Design review of the part built by this model. Coordinates are the model's own, in mm. Face numbers are marked on the shaded views. A direction names the side the tool comes from. Round coordinates to 2 decimals unless told otherwise and drop trailing zeros. Order: outer loops, then holes, each group sorted by start corner. A loop starts at its lowest first (then second) coordinate and runs counter-clockwise, first axis right, second up.
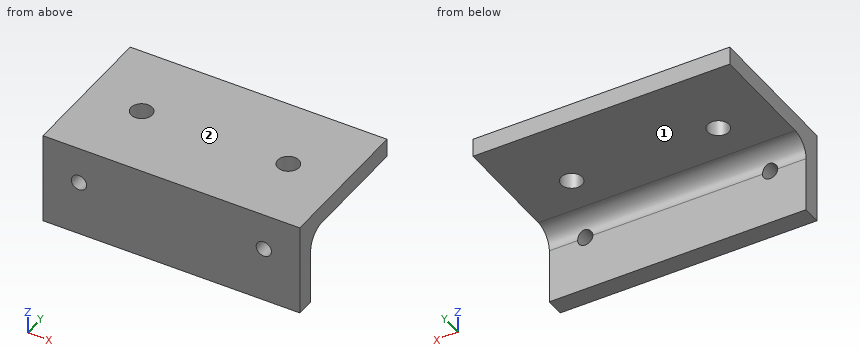
Autodesk Inventor part; units mm, degrees
ref_plane "YZ Plane" through (0, 0, 0) normal (1, 0, 0) x (0, 1, 0)
ref_plane "XZ Plane" through (0, 0, 0) normal (0, 1, 0) x (-1, 0, 0)
ref_plane "XY Plane" through (0, 0, 0) normal (0, 0, 1) x (1, 0, 0)
sketch "Sketch1" plane through (0, 0, 0) normal (1, 0, 0) x (0, 1, 0)
  line L0 (0, 0) -> (25.4, 0)
  line L1 (25.4, 0) -> (25.4, -3.175)
  line L2 (25.4, -3.175) -> (3.175, -3.175)
  line L3 (3.175, -3.175) -> (3.175, -15.875)
  line L4 (3.175, -15.875) -> (0, -15.875)
  line L5 (0, -15.875) -> (0, 0)
  dimension "d0" = 25.4
  dimension "d2" = 3.175
  dimension "d21" = 15.875
extrude "Extrusion1" add sketch "Sketch1" along normal mid plane 44.45
fillet "Fillet1" radius 3.175 1 edges at (0, 3.175, -3.175)
sketch "Sketch2" plane through (-22.225, 0, -15.875) normal (0, -1, 0) x (1, 0, 0)
  line L0 (38.225, 9.525) -> (6.225, 9.525) construction
  line L1 (0, 15.875) -> (44.45, 15.875) construction
  point P0 (22.225, 15.875)
  point P1 (22.225, 9.525)
  point P2 (22.225, 15.875)
  dimension "d6" = 6.35
  dimension "d7" = 32
hole "Hole1" at (16, 0, -6.35) at (-16, 0, -6.35) direction (0, 1, 0) diameter 2.6416 end through all
sketch "Sketch3" plane through (-22.225, 0, 0) normal (0, 0, 1) x (1, 0, 0)
  line L0 (0, 0) -> (44.45, 0) construction
  line L1 (0, 25.4) -> (44.45, 25.4) construction
  line L2 (34.925, 12.7) -> (9.525, 12.7) construction
  point P0 (22.225, 0)
  point P1 (22.225, 0)
  point P2 (22.225, 12.7)
  point P3 (22.225, 0)
  dimension "d15" = 25.4
  dimension "d22" = 12.7
hole "Hole2" at (12.7, 12.7, 0) at (-12.7, 12.7, 0) direction (0, 0, -1) diameter 3.683 end through all
properties part number "GP7-005" material "Aluminum 6061"
1) To check wall thickness, follow line 1 along X through (y, z) = (1.2, -6.35) (3 decimals); line 2 along X through (y, z) = (12.7, -0.95) (1 decimal); line 3 along Y through (x, z) = (12.7, -1.55). State the ranges of each line that lie inside material, in increasing order.
Results:
line 1: x = -22.225 to -17.321, -14.679 to 14.679, 17.321 to 22.225
line 2: x = -22.2 to -14.5, -10.9 to 10.9, 14.5 to 22.2
line 3: y = 0 to 10.86, 14.54 to 25.4
2) Clearance check with flat-ended pins moving along their axes: P1, Ø8, axis at y = 22, z = -11, coming from the +X side; P2, Ø3, axis at x = 16, z = -6.35, coming from the +Y side; P3, Ø1.5, axis at x = 14, y = 10, coming from the -Z side (3 decimals). State where each tip first meets the part, or that it passes through.
Results:
P1: passes through
P2: stops at y = 3.55
P3: stops at z = -3.175
3) Take a section at A-A on y = 12.7. Give the boundary of the cut face in (x, z) (1 decimal).
Results:
outline: (-22.2, -3.2) - (-14.5, -3.2) - (-14.5, 0) - (-22.2, 0) - close; (-10.9, -3.2) - (10.9, -3.2) - (10.9, 0) - (-10.9, 0) - close; (14.5, -3.2) - (22.2, -3.2) - (22.2, 0) - (14.5, 0) - close
4) Take a section at D-D on y = 2. Give the boundary of the cut face in (x, z) (3 decimals).
Results:
outline: (-22.225, -15.875) - (22.225, -15.875) - (22.225, 0) - (-22.225, 0) - close; hole circle Ø2.642 at (-16, -6.35); hole circle Ø2.642 at (16, -6.35)
5) Take a section at C-C on x = 5. Give the boundary of the cut face in (y, z) (3 decimals).
Results:
outline: (0, -15.875) - (3.175, -15.875) - (3.175, -6.35) arc R3.175 cw to (6.35, -3.175) - (25.4, -3.175) - (25.4, 0) - (0, 0) - close
6) For the marked faces 1 and 2, list the 3-axis set-ups (+Z, -Z, +X, -X, +Y, -Y) from which the entire face can be reached by the end or side of a thin tool; tool diameter is ignored.
Results:
face 1: -Z, +X, -X, +Y
face 2: +Z, +X, -X, +Y, -Y
